from build123d import *

# Parameters (mm, degrees)
F0_R     = 3.3686848121
F0_R_2   = 3.7503411647
F1_DEPTH = 25.4


# Not quite as in the source:
# - the program builds the solid bodies; features that only make, move or delete a surface that nothing else refers to are left out


with BuildPart() as f1:
    # F0 (on Top) → F1 (new body)
    with BuildSketch(Plane.XY):
        with BuildLine():
            Line((-11.4056267505, -5.9082075022), (-11.4056267505, 38.28210113))
            ThreePointArc((-11.4056267505, 38.28210113), (-13.0902542949, 40.0050046024), (-14.9420781413, 41.5467940758))
            ThreePointArc((-14.9420781413, 41.5467940758), (-24.4960295494, 45.8046369765), (-34.9515650706, 45.5063239844))
            ThreePointArc((-34.9515650706, 45.5063239844), (-41.3833712338, 42.777482568), (-46.7318524877, 38.28210113))
            Line((-46.7318524877, 38.28210113), (-46.7318524877, 22.8735643321))
            Line((-46.7318524877, 22.8735643321), (-37.9002960534, 22.7850040211))
            Line((-37.9002960534, 22.7850040211), (-33.5099794506, 22.7409791874))
            Line((-33.5099794506, 22.7409791874), (-29.0687396191, 22.6964437101))
            ThreePointArc((-29.0687396191, 22.6964437101), (-32.3476402886, 2.6663309949), (-30.4037962217, -17.5370864196))
            ThreePointArc((-30.4037962217, -17.5370864196), (-28.3292963567, -17.9171307498), (-27.2098111607, -19.7045132715))
            ThreePointArc((-27.2098111607, -19.7045132715), (-22.8158840867, -19.1811881286), (-19.9977839656, -22.5927531719))
            ThreePointArc((-19.9977839656, -22.5927531719), (-19.0499304153, -22.7087900697), (-18.1556105797, -23.043577982))
            Line((-18.1556105797, -23.043577982), (-11.4056267505, -22.5927531719))
            Line((-11.4056267505, -22.5927531719), (-11.4056267505, -14.6515189691))
            ThreePointArc((-11.4056267505, -14.6515189691), (-0.2868217682, -14.1752443759), (7.1637327783, -5.9082075022))
            ThreePointArc((7.1637327783, -5.9082075022), (7.197230267, 3.2378107083), (11.5452415215, 11.2842738641))
            ThreePointArc((11.5452415215, 11.2842738641), (1.5408183988, 7.0311325334), (0, -3.7300742697))
            ThreePointArc((0, -3.7300742697), (-5.7908190197, -4.3583061138), (-11.4056267505, -5.9082075022))
        make_face()
        Polygon((-25.470810011, 0), (-16.5671050976, 1.5869429488), (-20.5766428262, -8.2222158089), align=None, mode=Mode.SUBTRACT)
        with Locations((-40.4367111623, 32.953761518)):
            Circle(F0_R, mode=Mode.SUBTRACT)
        with Locations((-29.0687396191, 32.953761518)):
            Circle(F0_R_2, mode=Mode.SUBTRACT)
        with BuildLine():
            Line((-37.9002960534, 22.7850040211), (-46.7318524877, 22.8735643321))
            ThreePointArc((-46.7318524877, 22.8735643321), (-53.4771270799, 0.7607999274), (-45.7492200512, -21.028016743))
            ThreePointArc((-45.7492200512, -21.028016743), (-44.0238078591, -20.1849073614), (-42.104174186, -20.131174475))
            ThreePointArc((-42.104174186, -20.131174475), (-40.558011078, -20.7291440142), (-39.3299119733, -21.8426791577))
            ThreePointArc((-39.3299119733, -21.8426791577), (-39.2808229847, -18.7066363859), (-36.8050348739, -16.7811112041))
            ThreePointArc((-36.8050348739, -16.7811112041), (-39.1633371869, 2.951823761), (-37.9002960534, 22.7850040211))
        make_face()
        with BuildLine():
            ThreePointArc((-42.104174186, -20.131174475), (-44.0238078591, -20.1849073614), (-45.7492200512, -21.028016743))
            ThreePointArc((-45.7492200512, -21.028016743), (-46.9337681485, -22.4383900317), (-47.4600126918, -24.2034321528))
            ThreePointArc((-47.4600126918, -24.2034321528), (-44.2480891567, -28.8954606668), (-38.8667027357, -27.059088003))
            ThreePointArc((-38.8667027357, -27.059088003), (-34.3322542596, -30.4586049869), (-29.7978057834, -27.059088003))
            ThreePointArc((-29.7978057834, -27.059088003), (-27.4071947516, -31.3060964302), (-22.8805579245, -29.5000895858))
            ThreePointArc((-22.8805579245, -29.5000895858), (-16.7448352708, -29.0331395554), (-18.1556105797, -23.043577982))
            ThreePointArc((-18.1556105797, -23.043577982), (-19.0499304153, -22.7087900697), (-19.9977839656, -22.5927531719))
            ThreePointArc((-19.9977839656, -22.5927531719), (-22.8158840867, -19.1811881286), (-27.2098111607, -19.7045132715))
            ThreePointArc((-27.2098111607, -19.7045132715), (-28.3292963567, -17.9171307498), (-30.4037962217, -17.5370864196))
            ThreePointArc((-30.4037962217, -17.5370864196), (-31.8655744774, -18.4799458919), (-32.4125880239, -20.131174475))
            ThreePointArc((-32.4125880239, -20.131174475), (-32.5829263413, -19.4613489943), (-32.7484000877, -18.7903052132))
            ThreePointArc((-32.7484000877, -18.7903052132), (-34.4248384474, -17.0752518162), (-36.8050348739, -16.7811112041))
            ThreePointArc((-36.8050348739, -16.7811112041), (-39.2808229847, -18.7066363859), (-39.3299119733, -21.8426791577))
            ThreePointArc((-39.3299119733, -21.8426791577), (-40.558011078, -20.7291440142), (-42.104174186, -20.131174475))
        make_face()
        with BuildLine():
            ThreePointArc((-38.8667027357, -22.5927531719), (-39.1211782585, -22.231840123), (-39.3299119733, -21.8426791577))
            ThreePointArc((-39.3299119733, -21.8426791577), (-39.0800443488, -22.2064378205), (-38.8667027357, -22.5927531719))
        make_face(mode=Mode.SUBTRACT)
    extrude(amount=F1_DEPTH)


solid = f1.part
The listing builds one solid part. Answer for the finished solid, in the listing's coordinates (mm). A direction names the side the tool comes from. Give positions to 0.01 mm unless a question says otherwise; leave off trailing zeros. Write each loop counter-clockwise with the first axis right and the second up, starting at its lowest first coordinate (ties: lowest second). Pieces come first, ordered by that corner, then holes.
1) Section A-A (x = -19) is taken. Write down the section's boundary in (y, z).
2) Section D-D (x = -6) is taken. Write down the section's boundary in (y, z).
3) For a pull along X with two mould halves and no side action, classify faces 1 (the face through (-29, 8, 25.4)), 2 (the face through (-46.732, 31, 13)), 3 (the face through (-32.338, 2.951, 12.522)) as pulls with the +X half, pulls with the -X half, needs draft (parallel to the pull), parting line crosses it, or undercut.
4) Find the intervals of material crossed by L1, parallel to X at y = 9.5, z = 18; L2, parallel to X at y = 8, z = 2.5; L3, parallel to X at y = 22.5, z = 12.5, in increasing order.
5) Section B-B (y = 20) is taken. Write down the section's boundary in (x, z).
6) Section C-C (z = 23) is taken. Write down the section's boundary in (x, y) (1 decimal), and give its area (3 significant figures).
7) Given P1, Ø8, axis at y = 17.5, z = 22, coming from the -X side; P2, Ø2, axis at x = -23.5, z = 14.5, coming from the +Y side; P3, Ø8, axis at x = -41, z = 18.5, coming from the +Y side; P4, Ø4.5, axis at x = -29.07, y = 32.95, coming from the -Z side, each flat-ended and moving along its own axis, determine where each tip first touches the part or whether it passes through.
8) A tool of negligible diameter and unlimited length cuts with its end or side. For faces 4 (the face through (7.166, 3.112, 12.522)), 5 (the face through (-11.406, 16, 13)), 6 (the face through (-34.394, -17.091, 12.522)), from which of +Z, -Z, +X, -X, +Y, -Y can it reach the whole face along a straight path? Write none if from no direction.
Response:
1. outline: (-30.56, 0) - (-4.37, 0) - (-4.37, 25.4) - (-30.56, 25.4) - close; (1.15, 0) - (43.99, 0) - (43.99, 25.4) - (1.15, 25.4) - close
2. outline: (-15.54, 0) - (-4.4, 0) - (-4.4, 25.4) - (-15.54, 25.4) - close
3. face 1: needs draft
3. face 2: pulls with the -X half
3. face 3: undercut
4. L1: x = -52.63 to -39.15, -31.82 to -11.41, 4.18 to 10.1
4. L2: x = -52.93 to -39.19, -31.99 to -11.41, 2.38 to 9.14
4. L3: x = -46.99 to -37.94, -29.13 to -11.41
5. outline: (-48.57, 0) - (-38.3, 0) - (-38.3, 25.4) - (-48.57, 25.4) - close; (-29.83, 0) - (-11.41, 0) - (-11.41, 25.4) - (-29.83, 25.4) - close
6. outline: (-47.5, -24.2) arc R4.7 ccw to (-38.9, -27.1) arc R4.7 ccw to (-29.8, -27.1) arc R3.7 ccw to (-22.9, -29.5) arc R4 ccw (long way) to (-18.2, -23) - (-11.4, -22.6) - (-11.4, -14.7) arc R14.4 ccw to (7.2, -5.9) arc R18.8 cw to (11.5, 11.3) arc R11.1 ccw to (0, -3.7) arc R36.2 ccw to (-11.4, -5.9) - (-11.4, 38.3) arc R23.6 ccw to (-46.7, 38.3) - (-46.7, 22.9) arc R36.9 ccw to (-45.7, -21) arc R4.5 ccw to start; hole circle Ø6.7 at (-40.4, 33); hole (-39.3, -21.8) arc R3.6 ccw to (-38.9, -22.6) arc R4.5 ccw to start; hole (-37.9, 22.8) arc R109 ccw to (-36.8, -16.8) arc R3.6 cw to (-32.7, -18.8) arc R95.3 ccw to (-32.4, -20.1) arc R2.6 cw to (-30.4, -17.5) arc R78.8 cw to (-29.1, 22.7) - close; hole circle Ø7.5 at (-29.1, 33); hole (-25.5, 0) - (-20.6, -8.2) - (-16.6, 1.6) - close
6. area: 2,630 mm2
7. P1: stops at x = -51.51
7. P2: stops at y = 45.81
7. P3: stops at y = 44.88
7. P4: passes through
8. face 4: +Z, -Z, +X
8. face 5: +Z, -Z, +Y
8. face 6: +Z, -Z
